from build123d import *

# Parameters (mm, degrees)
F0_W     = 25.4
F0_H     = 127
F1_DEPTH = 12.7
F3_DEPTH = 17.78
F5_DEPTH = 25.4
F6_R     = 5.07999


# Not quite as in the source:
# - a fillet or chamfer is up to 0.001 mm smaller than in the source, because OpenCascade refuses the exact size


with BuildPart() as f1:
    # F0 (on Front) → F1 (new body)
    with BuildSketch(Plane.XZ):
        with Locations((12.7, 63.5)):
            Rectangle(F0_W, F0_H)
        Polygon((25.4, 0), (0, 0), (0, -25.4), (330.2, -25.4), (330.2, 0), align=None)
    extrude(amount=F1_DEPTH)

    # F2 (on face) → F3 (join)
    with BuildSketch(Plane.XZ.offset(12.7)):
        with BuildLine():
            ThreePointArc((12.7, 121.92), (7.3118463274, 108.9118463274), (20.32, 114.3))
            ThreePointArc((20.32, 114.3), (18.0881536726, 119.6881536726), (12.7, 121.92))
        make_face()
    extrude(amount=F3_DEPTH)

    # F4 (on face) → F5 (cut)
    with BuildSketch(Plane.XZ.offset(12.7)):
        Polygon((82.423, 3.81), (82.423, 0), (84.328, 0), (86.233, 0), (86.233, 3.81), align=None)
        Polygon((84.328, 0), (82.423, 0), (82.423, -3.81), (86.233, -3.81), (86.233, 0), align=None)
        Polygon((302.895, 3.81), (302.895, 0), (302.895, -3.81), (306.705, -3.81), (306.705, 3.81), align=None)
        Polygon((275.209, 3.81), (275.209, 0), (277.114, 0), (279.019, 0), (279.019, 3.81), align=None)
        Polygon((277.114, 0), (275.209, 0), (275.209, -3.81), (279.019, -3.81), (279.019, 0), align=None)
        Polygon((247.015, 3.81), (247.015, 0), (248.92, 0), (250.825, 0), (250.825, 3.81), align=None)
        Polygon((248.92, 0), (247.015, 0), (247.015, -3.81), (250.825, -3.81), (250.825, 0), align=None)
        Polygon((218.059, 3.81), (218.059, 0), (219.964, 0), (221.869, 0), (221.869, 3.81), align=None)
        Polygon((219.964, 0), (218.059, 0), (218.059, -3.81), (221.869, -3.81), (221.869, 0), align=None)
        Polygon((188.087, 3.81), (188.087, 0), (189.992, 0), (191.897, 0), (191.897, 3.81), align=None)
        Polygon((189.992, 0), (188.087, 0), (188.087, -3.81), (191.897, -3.81), (191.897, 0), align=None)
        Polygon((156.591, 3.81), (156.591, 0), (158.496, 0), (160.401, 0), (160.401, 3.81), align=None)
        Polygon((158.496, 0), (156.591, 0), (156.591, -3.81), (160.401, -3.81), (160.401, 0), align=None)
        Polygon((122.555, 3.81), (122.555, 0), (124.46, 0), (126.365, 0), (126.365, 3.81), align=None)
        Polygon((124.46, 0), (122.555, 0), (122.555, -3.81), (126.365, -3.81), (126.365, 0), align=None)
    extrude(amount=-F5_DEPTH, mode=Mode.SUBTRACT)

    # F6 (radius 5.08 in the source; OpenCascade refuses exactly that, so slightly less here)
    f6_edges = [f1.edges().sort_by_distance(p)[0] for p in [
        (165.1, -12.7, -25.4),
        (165.1, 0, -25.4),
        (0, 0, 50.8),
        (0, -12.7, 50.8),
        (12.7, 0, 127),
        (12.7, -12.7, 127),
        (25.4, 0, 63.5),
        (25.4, -12.7, 63.5),
        (330.2, 0, -12.7),
        (330.2, -12.7, -12.7),
    ]]
    fillet(f6_edges, radius=F6_R)


solid = f1.part
Here's how the part is built. I have some questions about the finished solid (model axes, mm). A direction names the side the tool comes from. Coordinates: 2 decimals unless noted, no trailing zeros. Loops run counter-clockwise (first coordinate to the right, second up) from the corner with the lowest first, then second, coordinate; pieces in that order, holes last.
1. For faces 1 (the flat face through (319, -6, 0)), 2 (the flat face through (129, 0, -2)), which set-ups out of +Z, -Z, +X, -X, +Y, -Y let a thin tool reach every point of the face, with its end or its side?
2. Imagine slicing it at B-B, the plane x = 74. Please give me the cut outline in (y, z).
3. Imagine slicing it at A-A, the plane z = 56. Please give me the cut outline in (x, y), and give its area (3 significant figures).
4. Imagine slicing it at C-C, the plane y = -16.5. Please give me the cut outline in (x, z), and give its area (3 significant figures).
5. For P1, Ø10, axis at x = 204.5, y = -9.5, coming from the +Z side; P2, Ø1.9, axis at x = 124.5, y = -5, coming from the +Z side; P3, Ø5, axis at x = 259.5, y = -14, coming from the -Z side, each with a flat end and sliding along its axis, tell me the tip position at first contact or that it passes through.
6. I need wall thicknesses on L1, parallel to Y at x = 54, z = -5; L2, parallel to X at y = -4.5, z = 48; L3, parallel to Z at x = 290.5, y = -10.5. Which ranges of each line are inside material? Lowest first, please.
Taken from the geometry:
1. face 1: +Z, +X, +Y, -Y
1. face 2: +Z, -Z, +X, -X, +Y
2. outline: (-12.7, -20.32) arc R5.08 ccw to (-7.62, -25.4) - (-5.08, -25.4) arc R5.08 ccw to (0, -20.32) - (0, 0) - (-12.7, 0) - close
3. outline: (0, -7.62) arc R5.08 ccw to (5.08, -12.7) - (20.32, -12.7) arc R5.08 ccw to (25.4, -7.62) - (25.4, -5.08) arc R5.08 ccw to (20.32, 0) - (5.08, 0) arc R5.08 ccw to (0, -5.08) - close
3. area: 300 mm2
4. outline: circle Ø15.24 at (12.7, 114.3)
4. area: 182 mm2
5. P1: stops at z = 0
5. P2: stops at z = -3.81
5. P3: stops at z = -23.6
6. L1: y = -12.7 to 0
6. L2: x = 0.03 to 25.37
6. L3: z = -24.5 to 0
